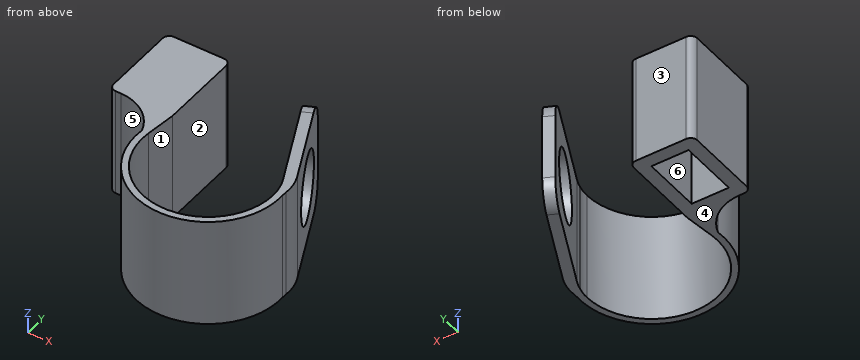
Autodesk Inventor part; units mm, degrees
ref_plane "YZ Plane" through (0, 0, 0) normal (1, 0, 0) x (0, 1, 0)
ref_plane "XZ Plane" through (0, 0, 0) normal (0, 1, 0) x (-1, 0, 0)
ref_plane "XY Plane" through (0, 0, 0) normal (0, 0, 1) x (1, 0, 0)
sketch "Sketch1" plane through (0, 0, 0) normal (0, 0, 1) x (1, 0, 0)
  line L0 (-0.85, -1.35) -> (0.85, -1.35)
  line L1 (0.85, -1.35) -> (0.85, 1.35)
  line L2 (0.85, 1.35) -> (-0.85, 1.35)
  line L3 (-0.85, 1.35) -> (-0.85, -1.35)
  line L4 (-0.85, -1.35) -> (0.85, 1.35) construction
  line L5 (0.85, -1.35) -> (-0.85, 1.35) construction
  line L6 (7.1105, -2.8923) -> (4.8846, 1.881)
  line L7 (4.8846, 1.881) -> (5.3378, 2.0923)
  line L8 (5.3378, 2.0923) -> (7.6622, -2.8923)
  line L9 (-1.45, 1.95) -> (1.45, 1.95)
  line L10 (1.45, 1.95) -> (1.45, -1.95)
  line L11 (1.148, -1.95) -> (-1.45, -1.95)
  line L12 (-1.45, -1.95) -> (-1.45, 1.95)
  line L13 (1.45, -1.95) -> (1.148, -1.95) construction
  line L14 (1.148, -1.95) -> (0.9806, -3.3133)
  line L15 (0.9806, -3.3133) -> (1.2826, -3.3133) construction
  line L16 (1.2826, -3.3133) -> (1.45, -1.95)
  line L17 (7.6622, -2.8923) -> (7.1105, -2.8923) construction
  line L18 (7.2357, -3.3923) -> (7.537, -3.3923) construction
  arc A0 (1.2826, -3.3133) -> (7.2357, -3.3923) centre (4.2548, -3.6783) ccw
  arc A1 (0.9806, -3.3133) -> (7.537, -3.3923) centre (4.2548, -3.6783) ccw
  line L19 (7.537, -3.3923) -> (7.6622, -2.8923)
  line L20 (7.1105, -2.8923) -> (7.2357, -3.3923)
  point P0 (0, 0)
  point P1 (6.5, -0.4)
  dimension "d0" = 1.7
  dimension "d1" = 2.7
  dimension "d4" = 0.5
  dimension "d5" = 5.5
  dimension "d16" = 0.6
  dimension "d17" = 0.6
  dimension "d18" = 0.6
  dimension "d19" = 0.6
  dimension "d20" = 25
  dimension "d21" = 6.5
  dimension "d22" = 0.3
  dimension "d25" = 0.5
  dimension "d38" = 83
  dimension "d39" = 0.4
extrude "Extrusion1" add sketch "Sketch1" along normal blind 5
fillet "Fillet1" radius 2 5 edges at (1.148, -1.95, 2.5) (7.537, -3.3923, 2.5) (7.6622, -2.8923, 2.5) (7.1105, -2.8923, 2.5) (7.2357, -3.3923, 2.5)
fillet "Fillet1" radius 0.3 3 edges at (-1.45, -1.95, 2.5) (-1.45, 1.95, 2.5) (1.45, 1.95, 2.5)
sketch "Sketch3" plane through (0, 0, 5) normal (0, 0, 1) x (1, 0, 0)
  line L0 (-0.85, 1.35) -> (0.85, 1.35)
  line L1 (-0.85, -1.35) -> (-0.85, 1.35)
  line L2 (0.85, 1.35) -> (0.85, -1.35)
  line L3 (0.85, -1.35) -> (-0.85, -1.35)
  point P0 (0, 0)
extrude "Extrusion3" add sketch "Sketch3" against normal blind 1
sketch "Sketch4" plane through (5.3378, 2.0923, 5) normal (0.9063078, 0.4226183, 0) x (0, 0, -1)
  line L0 (0, -4.8077) -> (5, 0) construction
  circle A0 centre (2.5, -2.4038) radius 1.5
  line L1 (0, -4.8077) -> (0, 0)
  line L2 (5, -4.8077) -> (5, 0)
  dimension "d33" = 3
extrude "Extrusion4" cut sketch "Sketch4" against normal up to surface (0.5 mm away)
fillet "Fillet3" radius 1 2 edges at (5.1112, 1.9867, 0) (5.1112, 1.9867, 5)
properties part number "ValveSpring"
Check sheet for the modelled part. Datum: model origin and axes. Units: mm. Face numbers are marked on the shaded views. A direction names the side the tool comes from. Round coordinates to 2 decimals unless told otherwise and drop trailing zeros. Loops run counter-clockwise (first coordinate to the right, second up) from the corner with the lowest first, then second, coordinate; pieces in that order, holes last. Notation, with made-up numbers: (52, 49.25) - (77, 49.25) arc R16 cw to (77, 74.25) - close; hole circle Ø6 at (22.5, -40). An arc over 180 degrees is marked (long way). Answer as a JSON object with one key per item and string values. Group by question number.
Q1. Mould release check, pull along X, two halves, no side actions. Record for the marked faces 4, 5 and 6: released by +X, released by -X, zero draft, split by the parting line, or undercut.
Q2. Sectioned sample at B-B, the plane y = -5.5. Enter the section's corners in (x, z).
Q3. Sectioned sample at C-C, the plane z = 0.8. Enter the section's corners in (x, y), plus the area to 3 significant figures.
Q4. Gauge pin test, flat ends, axial feed: P1, Ø2, axis at y = -0.5, z = 2, coming from the +X side; P2, Ø1.5, axis at y = -5, z = 0.5, coming from the +X side; P3, Ø1.9, axis at x = 0, y = -0.5, coming from the -Z side; P4, Ø1.2, axis at x = 0.5, z = 3, coming from the +Y side. Record the tip position at first contact, or that the pin passes through.
Q5. Sectioned sample at A-A, the plane z = 3.6. Enter the section's corners in (x, y).
Q6. Scan lines: line 1 along X through (y, z) = (0.5, 2.55); line 2 along X through (y, z) = (-0.75, 0.7); line 3 along Y through (x, z) = (5, 4). Record each from-to range of solid material in increasing order. Write a range as [from, to].
Q7. Set-up check for the marked faces 1, 2 and 3: record each of +Z, -Z, +X, -X, +Y, -Y from which the full face is reachable in a straight line by a thin tool's end or side.
Q8. Sectioned sample at D-D, the plane x = 0.5. Enter the section's corners in (y, z).
Solution:
{
 "1": {"face 4": "zero draft", "face 5": "released by -X", "face 6": "undercut"},
 "2": {"outline": "(1.51, 0) - (1.88, 0) - (1.88, 5) - (1.51, 5) - close; (6.63, 0) - (7, 0) - (7, 5) - (6.63, 5) - close"},
 "3": {"outline": "(-1.45, -1.65) arc R0.3 ccw to (-1.15, -1.95) - (-0.92, -1.95) arc R2 cw to (0.98, -3.31) arc R3.29 ccw (long way) to (7.55, -3.53) arc R2 cw to (7.55, -3.27) arc R2 ccw to (7.37, -2.26) - (5.35, 2.07) - (4.89, 1.86) - (7.03, -2.72) arc R2 cw to (7.16, -3.08) - (7.19, -3.21) arc R2 cw to (7.25, -3.72) arc R2.99 cw (long way) to (1.28, -3.31) - (1.45, -1.95) - (1.45, 1.65) arc R0.3 ccw to (1.15, 1.95) - (-1.15, 1.95) arc R0.3 ccw to (-1.45, 1.65) - close; hole (-0.85, -1.35) - (0.85, -1.35) - (0.85, 1.35) - (-0.85, 1.35) - close", "area": "13.9 mm²"},
 "4": {"P1": "stops at x = 7.01", "P2": "stops at x = 7.5", "P3": "stops at z = 0", "P4": "stops at y = 1.95"},
 "5": {"outline": "(-1.45, -1.65) arc R0.3 ccw to (-1.15, -1.95) - (-0.92, -1.95) arc R2 cw to (0.98, -3.31) arc R3.29 ccw (long way) to (7.55, -3.53) arc R2 cw to (7.55, -3.27) arc R2 ccw to (7.37, -2.26) - (6.78, -1.01) - (6.33, -1.22) - (7.03, -2.72) arc R2 cw to (7.16, -3.08) - (7.19, -3.21) arc R2 cw to (7.25, -3.72) arc R2.99 cw (long way) to (1.28, -3.31) - (1.45, -1.95) - (1.45, 1.65) arc R0.3 ccw to (1.15, 1.95) - (-1.15, 1.95) arc R0.3 ccw to (-1.45, 1.65) - close; (4.88, 1.88) - (5.47, 0.63) - (5.92, 0.84) - (5.34, 2.09) - close; hole (-0.85, -1.35) - (0.85, -1.35) - (0.85, 1.35) - (-0.85, 1.35) - close"},
 "6": {"line 1": "x = [-1.45, -0.85], [0.85, 1.45]", "line 2": "x = [-1.45, -0.85], [0.85, 1.45], [6.11, 6.66]", "line 3": "y = [-6.89, -6.58], [1.63, 1.93]"},
 "7": {"face 1": "+Z, -Z", "face 2": "+Z, -Z, +Y", "face 3": "+Z, -Z, -X, +Y"},
 "8": {"outline": "(-2.54, 0) - (-1.35, 0) - (-1.35, 4) - (1.35, 4) - (1.35, 0) - (1.95, 0) - (1.95, 5) - (-2.54, 5) - close"}
}
